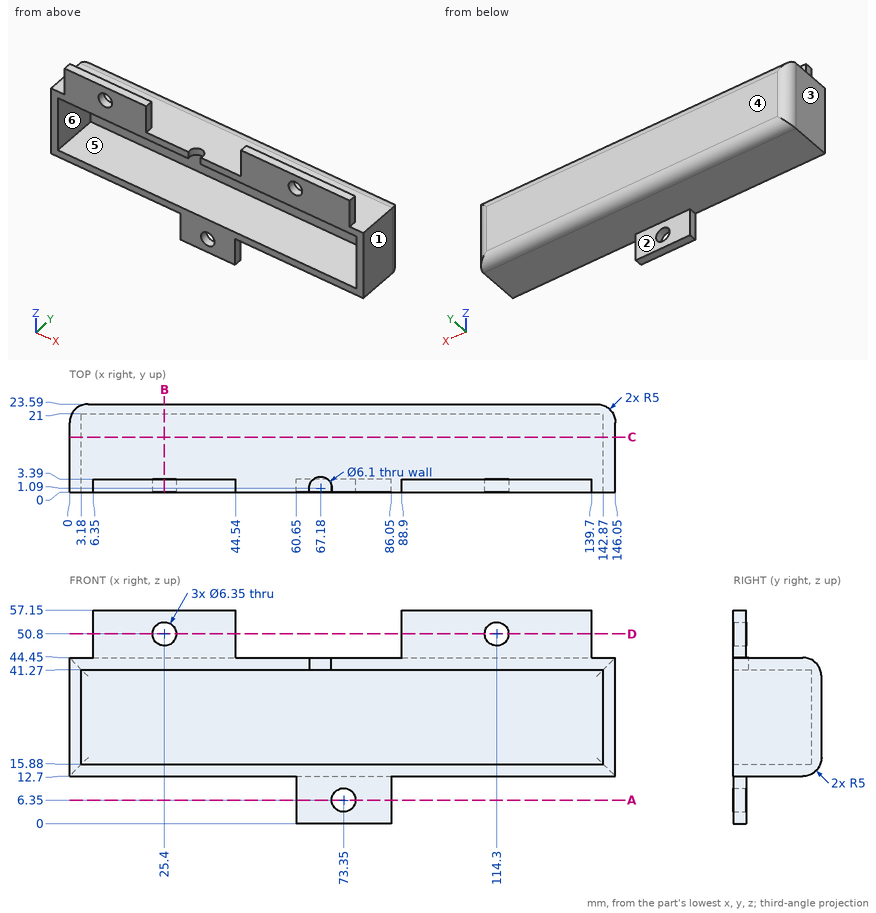
Geometry: see drawing. Coordinates: mm, zero at the bounding-box minimum. A direction names the side the tool comes from. Coordinates: 2 decimals unless noted, no trailing zeros. Loops run counter-clockwise (first coordinate to the right, second up) from the corner with the lowest first, then second, coordinate; pieces in that order, holes last. Notation, with made-up numbers: M 33.5,37 L 59.5,37 A17 cw 59.5,48 Z; hole C -14.75,88.5 d3. An arc over 180 degrees is marked long. Put each result on its own line as item: value. Start each with the question number.
1) Ray query, L1, parallel to Z at x = 73.35, y = 1.55 (3 decimals); L2, parallel to X at y = 2.55, z = 50.8 (3 decimals); L3, parallel to Z at x = 114.3, y = 1.45 (3 decimals). Return the intervals inside material, ascending. Write a range as from..to.
2) Contact query for flat-ended pins moving along their axis: pin 1 Ø2.5 at (y, z) = (2.5, 50.5) entering from +X; pin 2 Ø1 at (y, z) = (1.5, 53) entering from -X; pin 3 Ø8.5 at (x, z) = (114.3, 50.8) entering from +Y. Output: stop coordinate, or through.
3) Cut plane C-C on y = 14.75. Return the cut outline in (x, z), then the cut area to 3 significant figures.
4) Cut plane A-A on z = 6.35. Return the cut outline in (x, y) (3 decimals), then the cut area to 3 significant figures.
5) Reachability of the marked faces 1 and 2 from +Z, -Z, +X, -X, +Y, -Y: full face, straight path, thin tool, end or side. Return the list, or none.
6) Cut plane D-D on z = 50.8. Return the cut outline in (x, y) (3 decimals), then the cut area to 3 significant figures.
7) Pull-direction query (X, two-part tool) for the marked faces 3, 4, 5 and 6; classes: pulls with the +X half, pulls with the -X half, needs draft (parallel to the pull), parting line crosses it, or undercut.
8) Cut plane B-B on x = 25.4. Return the cut outline in (y, z) (3 decimals).
The answers:
1. L1: z = 0..3.175, 9.525..15.88, 41.27..44.45
1. L2: x = 6.35..22.225, 28.575..44.54, 88.9..111.125, 117.475..139.7
1. L3: z = 12.7..15.88, 41.27..47.625, 53.975..57.15
2. pin 1: stops at x = 139.7
2. pin 2: stops at x = 6.35
2. pin 3: stops at y = 3.39
3. outline: M 0,12.7 L 146.05,12.7 L 146.05,44.45 L 0,44.45 Z; hole M 3.18,15.88 L 142.87,15.88 L 142.87,41.27 L 3.18,41.27 Z
3. area: 1,090 mm²
4. outline: M 60.65,0 L 70.175,0 L 70.175,3.39 L 60.65,3.39 Z; M 76.525,0 L 86.05,0 L 86.05,3.39 L 76.525,3.39 Z
4. area: 64.6 mm²
5. face 1: +Z, -Z, +X, +Y, -Y
5. face 2: -Z, +X, -X, +Y
6. outline: M 6.35,0 L 22.225,0 L 22.225,3.39 L 6.35,3.39 Z; M 28.575,0 L 44.54,0 L 44.54,3.39 L 28.575,3.39 Z; M 88.9,0 L 111.125,0 L 111.125,3.39 L 88.9,3.39 Z; M 117.475,0 L 139.7,0 L 139.7,3.39 L 117.475,3.39 Z
6. area: 259 mm²
7. face 3: pulls with the -X half
7. face 4: needs draft
7. face 5: undercut
7. face 6: undercut
8. outline: M 0,12.7 L 18.59,12.7 A5 ccw 23.59,17.7 L 23.59,39.45 A5 ccw 18.59,44.45 L 3.39,44.45 L 3.39,47.625 L 0,47.625 L 0,41.27 L 21,41.27 L 21,15.88 L 0,15.88 Z; M 0,53.975 L 3.39,53.975 L 3.39,57.15 L 0,57.15 Z
